Work out the finished part from the listing and answer in its coordinate system (mm). A direction names the side the tool comes from. Give positions to 0.01 mm unless a question says otherwise; leave off trailing zeros. Order: outer loops, then holes, each group sorted by start corner. A loop starts at its lowest first (then second) coordinate and runs counter-clockwise, first axis right, second up. Notation, with made-up numbers: M 78,-37 L 120,-37 A28 cw 120,-17 Z; hole C -35.5,-36 d6. An arc over 180 degrees is marked long. One line per item, written item: value.
from build123d import *

# Parameters (mm, degrees)
SKETCH3_W           = 17.9
SKETCH3_H           = 11.9
BOSS_EXTRUDE3_DEPTH = 1.4
FILLET2_R           = 12
SKETCH4_W           = 19
SKETCH4_H           = 14
BOSS_EXTRUDE4_DEPTH = 1


with BuildPart() as part:
    # Sketch3 → Boss-Extrude3 (new body)
    with BuildSketch(Plane(origin=(0, 0, 0), x_dir=(1, 0, 0), z_dir=(0, 1, 0))):
        with Locations((19.738575208, -2.596225655)):
            Rectangle(SKETCH3_W, SKETCH3_H)
    extrude(amount=BOSS_EXTRUDE3_DEPTH)

    # Fillet2
    # the kernel refuses this fillet: 12 mm, written as the material it takes off along each edge
    with BuildSketch(Plane(origin=(10.788575208, -30, -3.353774345), x_dir=(1, 0, 0), z_dir=(0, 1, 0))) as fillet2_piece_1:
        with BuildLine():
            CenterArc((FILLET2_R, -FILLET2_R), FILLET2_R, 90, 90)
            Line((0, -FILLET2_R), (0, 0))
            Line((0, 0), (FILLET2_R, 0))
        make_face()
    extrude(amount=61.4, mode=Mode.SUBTRACT)
    with BuildSketch(Plane(origin=(28.688575208, -30, -3.353774345), x_dir=(-1, 0, 0), z_dir=(0, 1, 0))) as fillet2_piece_2:
        with BuildLine():
            CenterArc((FILLET2_R, FILLET2_R), FILLET2_R, 180, 90)
            Line((0, FILLET2_R), (0, 0))
            Line((0, 0), (FILLET2_R, 0))
        make_face()
    extrude(amount=61.4, mode=Mode.SUBTRACT)

    # Sketch4 → Boss-Extrude4 (add)
    with BuildSketch(Plane(origin=(0, 1.4, 0), x_dir=(1, 0, 0), z_dir=(0, 1, 0))):
        with Locations((19.738575208, -2.944154074)):
            Rectangle(SKETCH4_W, SKETCH4_H)
    extrude(amount=BOSS_EXTRUDE4_DEPTH)


solid = part.part
(1) Find the intervals of material crossed by probe 1 along Y at (x, z) = (28, -2.75); probe 2 along X at (y, z) = (1.1, 4); probe 3 along Z at (x, y) = (27, 0.2), in increasing order. Write a range as from..to.
Findings:
probe 1: y = 1.4..2.4
probe 2: x = 11.72..27.75
probe 3: z = 2.51..8.55
(2) Section C-C, the plane y = 0.35 is taken. Give the vertices of the cut face in (x, z), then the cut area to 3 significant figures.
Findings:
outline: M 10.79,8.55 A12 ccw 19.74,-2.96 A12 ccw 28.69,8.55 Z
area: 152 mm^2
(3) Which of the six approach directions +Z, -Z, +X, -X, +Y, -Y give full straight-line access (tool end or side, diameter ignored) to faces 1 (the cylindrical face through (13.384, 0.69, 1.192)), 2 (the flat face through (20, 1, 8.546)), 3 (the flat face through (20, 0, 4)), 4 (the cylindrical face through (26.23, 0.69, 1.37))?
Findings:
face 1: -Z, -X, -Y
face 2: +Z, +X, -X, -Y
face 3: +Z, -Z, +X, -X, -Y
face 4: -Z, +X, -Y
(4) Given P1, Ø4, axis at x = 22, z = 2, coming from the -Y side, flat-ended and moving along its own axis, determine where the tip first touches the part or whether it passes through.
Findings:
P1: stops at y = 0
(5) Section A-A, the plane z = 0 is taken. Give the vertices of the cut face in (x, y).
Findings:
outline: M 10.24,1.4 L 14.47,1.4 L 14.47,0 L 25.01,0 L 25.01,1.4 L 29.24,1.4 L 29.24,2.4 L 10.24,2.4 Z
(6) Section B-B, the plane x = 26.25 is taken. Give the vertices of the cut face in (y, z), then the cut area to 3 significant figures.
Findings:
outline: M 0,1.4 L 1.4,1.4 L 1.4,-4.06 L 2.4,-4.06 L 2.4,9.94 L 1.4,9.94 L 1.4,8.55 L 0,8.55 Z
area: 24.0 mm^2
